Part print with two shaded views. Sizes in mm from the minimum x, y, z corner. A direction names the side the tool comes from. Coordinates: 2 decimals unless noted, no trailing zeros. Order: outer loops, then holes, each group sorted by start corner. A loop starts at its lowest first (then second) coordinate and runs counter-clockwise, first axis right, second up. Notation, with made-up numbers: M 49,-19.75 L 84,-19.75 A26 ccw 84,2.25 Z; hole C 10.25,-18.75 d8. An arc over 180 degrees is marked long. Answer in a Markdown table with one row per item. Add a question column.
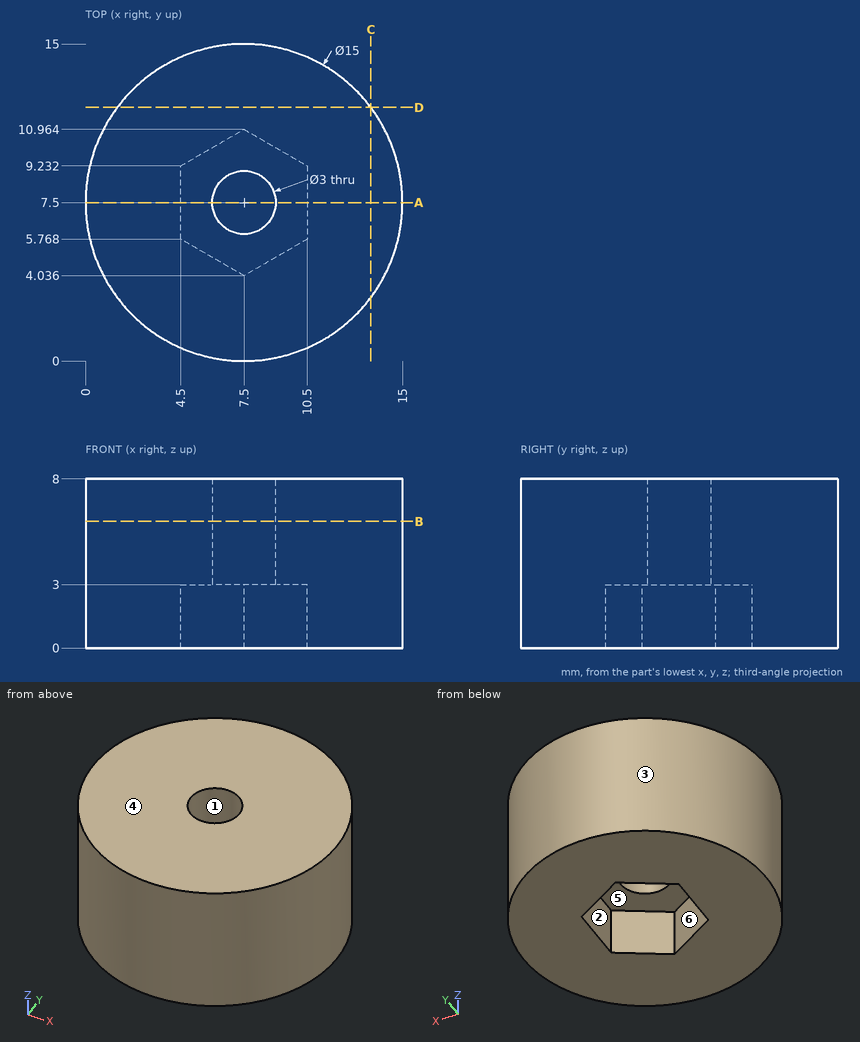
(1) Slice it at B-B (z = 6). List the corners of the cut face in (x, y).
(2) 3-axis set-ups, long thin cutter, end or side, ignore diameter. For the marked faces 1 and 2: which of +Z, -Z, +X, -X, +Y, -Y reach the whole face in a straight line?
(3) Pull direction X, two halves, no side cores. Call the marked faces 3, 4, 5 and 6: pulls with the +X half, pulls with the -X half, needs draft (parallel to the pull), parting line crosses it, or undercut.
(4) Wall check: line 1 (Y direction, x = 7.5, z = 5.3); line 2 (X direction, y = 8.25, z = 7); line 3 (X direction, y = 8.25, z = 0.75). Give the ranges that are in metal, low to high.
(5) Drop flat-ended pins along their axis: P1, Ø8, axis at x = 9, y = 11, coming from the -Z side; P2, Ø2, axis at x = 6, z = 4, coming from the +Y side; P3, Ø1.5, axis at y = 13.5, z = 3, coming from the +X side; P4, Ø1, axis at y = 4, z = 1.5, coming from the +X side. Give the stop position or say it passes through.
(6) Slice it at D-D (y = 12). List the corners of the cut face in (x, z), and give its area (3 significant figures).
(7) Slice it at A-A (y = 7.5). List the corners of the cut face in (x, z).
(8) Slice it at C-C (x = 13.5). List the corners of the cut face in (y, z), and give its area (3 significant figures).
Computed:
| question | item | result |
|---|---|---|
| 1 | outline | C 7.5,7.5 d15; hole C 7.5,7.5 d3 |
| 2 | face 1 | +Z, -Z |
| 2 | face 2 | -Z |
| 3 | face 3 | parting line crosses it |
| 3 | face 4 | needs draft |
| 3 | face 5 | undercut |
| 3 | face 6 | undercut |
| 4 | line 1 | y = 0 to 6, 9 to 15 |
| 4 | line 2 | x = 0.04 to 6.2, 8.8 to 14.96 |
| 4 | line 3 | x = 0.04 to 4.5, 10.5 to 14.96 |
| 5 | P1 | stops at z = 0 |
| 5 | P2 | stops at y = 14.98 |
| 5 | P3 | stops at x = 12.86 |
| 5 | P4 | stops at x = 14.37 |
| 6 | outline | M 1.5,0 L 13.5,0 L 13.5,8 L 1.5,8 Z |
| 6 | area | 96.0 mm^2 |
| 7 | outline | M 0,0 L 4.5,0 L 4.5,3 L 6,3 L 6,8 L 0,8 Z; M 9,3 L 10.5,3 L 10.5,0 L 15,0 L 15,8 L 9,8 Z |
| 8 | outline | M 3,0 L 12,0 L 12,8 L 3,8 Z |
| 8 | area | 72.0 mm^2 |
